Autodesk Inventor part; units mm, degrees
ref_plane "YZ Plane" through (0, 0, 0) normal (1, 0, 0) x (0, 1, 0)
ref_plane "XZ Plane" through (0, 0, 0) normal (0, 1, 0) x (-1, 0, 0)
ref_plane "XY Plane" through (0, 0, 0) normal (0, 0, 1) x (1, 0, 0)
sketch "Sketch1" plane through (0, 0, 0) normal (0, 0, 1) x (1, 0, 0)
  line L0 (17.0037, 144.1779) -> (514.0037, 144.1779)
  line L1 (514.0037, 144.1779) -> (514.0037, 949.1779)
  line L2 (514.0037, 949.1779) -> (17.0037, 949.1779)
  circle A0 centre (469.9509, 776.1779) radius 2.65
  circle A1 centre (469.9509, 899.1779) radius 2.65
  circle A2 centre (444.0037, 589.1779) radius 15
  circle A3 centre (444.0037, 619.1779) radius 1.5
  circle A4 centre (418.023, 574.1779) radius 1.5
  circle A5 centre (469.9845, 574.1779) radius 1.5
  line L3 (444.0037, 589.1779) -> (444.0037, 619.1779) construction
  line L4 (444.0037, 589.1779) -> (444.0037, 619.1779) construction
  line L5 (444.0037, 589.1779) -> (444.0037, 619.1779) construction
  line L6 (444.0037, 589.1779) -> (444.0037, 619.1779) construction
  line L7 (17.0037, 949.1779) -> (17.0037, 920.3279)
  line L8 (17.0037, 920.3279) -> (22.0037, 920.3279)
  line L9 (22.0037, 920.3279) -> (22.0037, 878.3279)
  line L10 (22.0037, 878.3279) -> (17.0037, 878.3279)
  line L11 (17.0037, 878.3279) -> (17.0037, 620.3279)
  line L12 (17.0037, 620.3279) -> (22.0037, 620.3279)
  line L13 (22.0037, 620.3279) -> (22.0037, 578.3279)
  line L14 (22.0037, 578.3279) -> (17.0037, 578.3279)
  line L15 (17.0037, 578.3279) -> (17.0037, 320.3279)
  line L16 (17.0037, 320.3279) -> (22.0037, 320.3279)
  line L17 (22.0037, 320.3279) -> (22.0037, 278.3279)
  line L18 (22.0037, 278.3279) -> (17.0037, 278.3279)
  line L19 (17.0037, 144.1779) -> (17.0037, 278.3279)
  line L20 (35.5037, 901.6779) -> (38.0037, 901.6779)
  line L21 (35.5037, 896.6779) -> (38.0037, 896.6779)
  arc A6 (35.5037, 901.6779) -> (35.5037, 896.6779) centre (35.5037, 899.1779) ccw
  arc A7 (38.0037, 896.6779) -> (38.0037, 901.6779) centre (38.0037, 899.1779) ccw
  line L22 (35.5037, 601.6779) -> (38.0037, 601.6779)
  line L23 (35.5037, 596.6779) -> (38.0037, 596.6779)
  line L24 (35.5037, 301.6779) -> (38.0037, 301.6779)
  line L25 (35.5037, 296.6779) -> (38.0037, 296.6779)
  arc A8 (35.5037, 301.6779) -> (35.5037, 296.6779) centre (35.5037, 299.1779) ccw
  arc A9 (38.0037, 296.6779) -> (38.0037, 301.6779) centre (38.0037, 299.1779) ccw
  arc A10 (35.5037, 601.6779) -> (35.5037, 596.6779) centre (35.5037, 599.1779) ccw
  arc A11 (38.0037, 596.6779) -> (38.0037, 601.6779) centre (38.0037, 599.1779) ccw
  dimension "d72" = 497
  dimension "d73" = 805
  dimension "d85" = 50
  dimension "d133" = 5.3
  dimension "d134" = 5.3
  dimension "d135" = 123
  dimension "d168" = 50
  dimension "d218" = 30
  dimension "d219" = 70
  dimension "d221" = 3
  dimension "d222" = 3
  dimension "d223" = 3
  dimension "d224" = 30
  dimension "d228" = 15
  dimension "d230" = 15
  dimension "d231" = 25.9808
  dimension "d232" = 25.9808
  dimension "d233" = 360
  dimension "d248" = 300
  dimension "d249" = 300
  dimension "d250" = 28.85
  dimension "d251" = 5
  dimension "d252" = 42
  dimension "d253" = 90
  dimension "d254" = 5
  dimension "d255" = 90
  dimension "d256" = 21
  dimension "d257" = 5
  dimension "d258" = 42
  dimension "d259" = 5
  dimension "d260" = 90
  dimension "d261" = 5
  dimension "d262" = 90
  dimension "d263" = 42
  dimension "d264" = 90
  dimension "d265" = 5
  dimension "d266" = 90
  dimension "d268" = 258
  dimension "d269" = 258
  dimension "d270" = 2.5
  dimension "d271" = 5
  dimension "d272" = 7.5
  dimension "d273" = 5
  dimension "d274" = 7.5
  dimension "d275" = 2.5
  dimension "d276" = 7.5
  dimension "d277" = 2.5
  dimension "d278" = 5
extrude "Extrusion2" add sketch "Sketch1" along normal blind 3 contours L19 L18 L17 L16 L15 L14 L13 L12 L11 L10 L9 L8 L7 L2 L1 L0 | A0 | A1 | A2 | A3 | A4 | A5 | L20 A7 L21 A6 | L22 A11 L23 A10 | L24 A9 L25 A8
hole "Hole7" at (38.0037, 899.1779, 0) direction (0, 0, 1) diameter 5 end through all
hole "Hole8" at (38.0037, 599.1779, 0) direction (0, 0, 1) diameter 5 end through all
hole "Hole9" at (38.0037, 299.1779, 0) direction (0, 0, 1) diameter 5 end through all
hole "Hole13" at (469.9509, 776.1779, 0) direction (0, 0, 1) diameter 5.3 end through all
hole "Hole14" at (469.9509, 899.1779, 0) direction (0, 0, 1) diameter 5.3 end through all
extrude "Extrusion7" cut sketch "Sketch1" along normal blind 10 contours A2
extrude "Extrusion8" cut sketch "Sketch1" along normal blind 10 contours A3
extrude "Extrusion9" cut sketch "Sketch1" along normal blind 10 contours A4
extrude "Extrusion10" cut sketch "Sketch1" along normal blind 10 contours A5
equation "\"d91\" = d81"
equation "\"d98\" = d81"
equation "\"d105\" = d81"
equation "\"d137\" = d133"
equation "\"d144\" = d133"
properties part number "Plexiglas_Einfassung_550x710mm" material "Polycarbonate, Clear"
Model file for the job. Use its own axes, mm. Give positions to 0.01 mm unless a question says otherwise; leave off trailing zeros.
Item 1: Drill centre lines: line 1 along X through (y, z) = (913.5, 0.7); line 2 along X through (y, z) = (298, 2.45). Where is each one in solid material? Low to high.
Check values:
line 1: x = 22 to 514
line 2: x = 22 to 35.8, 40.21 to 514
Item 2: Mould opens along X. For faces 1 (the face through (457.86, 594.92, 1.48)), 2 (the face through (262, 552, 0)) say: +X half, -X half, draft (parallel to the pull), parting line (faces both ways), or undercut.
Check values:
face 1: undercut
face 2: draft
Item 3: Drop flat-ended pins along their axis: P1, Ø1.5, axis at y = 904.5, z = 1, coming from the -X side; P2, Ø5, axis at x = 469.95, y = 899.18, coming from the -Z side. Give the stop position or say it passes through.
Check values:
P1: stops at x = 22
P2: passes through
